Input: part model. Units: mm. Frame: model coordinates. A direction names the side the tool comes from. Give positions to 0.01 mm unless a question says otherwise; leave off trailing zeros. Loops run counter-clockwise (first coordinate to the right, second up) from the corner with the lowest first, then second, coordinate; pieces in that order, holes last. Notation, with made-up numbers: (62, -4.5) - (100, -4.5) arc R20 cw to (100, 5.5) - close; hole circle Ø7 at (68, -24.5). An arc over 180 degrees is marked (long way). Answer as a JSON object with one key per item and string values.
from build123d import *

# Parameters (mm, degrees)
MODEL_R             = 1.6
MODEL_R_2           = 2
BOSS_EXTRUDE1_DEPTH = 10


with BuildPart() as part:
    # Model → Boss-Extrude1 (new body)
    with BuildSketch(Plane.XY):
        Polygon((85, 428), (85, 0), (-85, 0), (-85, 428), (-77, 436), (77, 436), align=None)
        with Locations((-31.5, 50)):
            Circle(MODEL_R, mode=Mode.SUBTRACT)
        with Locations((-31.5, 30)):
            Circle(MODEL_R, mode=Mode.SUBTRACT)
        with Locations((31.5, 30)):
            Circle(MODEL_R, mode=Mode.SUBTRACT)
        with Locations((31.5, 50)):
            Circle(MODEL_R, mode=Mode.SUBTRACT)
        with Locations((-58, 50)):
            Circle(MODEL_R, mode=Mode.SUBTRACT)
        with Locations((-73, 210)):
            Circle(MODEL_R_2, mode=Mode.SUBTRACT)
        with Locations((-73, 230)):
            Circle(MODEL_R_2, mode=Mode.SUBTRACT)
        with Locations((60, 355)):
            Circle(MODEL_R, mode=Mode.SUBTRACT)
        with Locations((58, 50)):
            Circle(MODEL_R, mode=Mode.SUBTRACT)
        with Locations((-60, 355)):
            Circle(MODEL_R, mode=Mode.SUBTRACT)
        with Locations((-28, 355)):
            Circle(MODEL_R, mode=Mode.SUBTRACT)
        with Locations((28, 355)):
            Circle(MODEL_R, mode=Mode.SUBTRACT)
        with Locations((60, 5)):
            Circle(MODEL_R, mode=Mode.SUBTRACT)
        with Locations((28, 5)):
            Circle(MODEL_R, mode=Mode.SUBTRACT)
        with Locations((-28, 5)):
            Circle(MODEL_R, mode=Mode.SUBTRACT)
        with Locations((-60, 5)):
            Circle(MODEL_R, mode=Mode.SUBTRACT)
        with Locations((10, 375)):
            Circle(MODEL_R, mode=Mode.SUBTRACT)
        with Locations((-10, 375)):
            Circle(MODEL_R, mode=Mode.SUBTRACT)
        with BuildLine():
            Line((14, 34.5), (20, 34.5))
            ThreePointArc((20, 34.5), (21.414213562, 33.914213562), (22, 32.5))
            Line((22, 32.5), (22, 14.5))
            ThreePointArc((22, 14.5), (21.414213562, 13.085786438), (20, 12.5))
            Line((20, 12.5), (14, 12.5))
            ThreePointArc((14, 12.5), (12.585786438, 13.085786438), (12, 14.5))
            Line((12, 14.5), (12, 32.5))
            ThreePointArc((12, 32.5), (12.585786438, 33.914213562), (14, 34.5))
        make_face(mode=Mode.SUBTRACT)
        Polygon((-29, 315), (29, 315), (35, 309), (35, 61), (29, 55), (-29, 55), (-35, 61), (-35, 309), align=None, mode=Mode.SUBTRACT)
        with BuildLine():
            Line((-54, 392), (-54, 412))
            ThreePointArc((-54, 412), (-52.242640687, 416.242640687), (-48, 418))
            Line((-48, 418), (48, 418))
            ThreePointArc((48, 418), (52.242640687, 416.242640687), (54, 412))
            Line((54, 412), (54, 392))
            ThreePointArc((54, 392), (52.242640687, 387.757359313), (48, 386))
            Line((48, 386), (-48, 386))
            ThreePointArc((-48, 386), (-52.242640687, 387.757359313), (-54, 392))
        make_face(mode=Mode.SUBTRACT)
    extrude(amount=BOSS_EXTRUDE1_DEPTH)


solid = part.part
Item 1: Cut plane C-C (y = 406.5). Return loops of the section in (x, z), then the cut area to 3 significant figures.
Geometry check:
{"outline": "(-85, 0) - (-54, 0) - (-54, 10) - (-85, 10) - close; (54, 0) - (85, 0) - (85, 10) - (54, 10) - close", "area": "620 mm2"}
Item 2: Mould query, pull axis Y, two halves, no side actions, for faces 3 (the face through (-1, 418, 5)), 4 (the face through (-1, 436, 5)), 5 (the face through (-85, 211, 5)), 6 (the face through (35, 187, 5)). Classes: released by +Y, released by -Y, zero draft, split by the parting line, or undercut.
Geometry check:
{"face 3": "undercut", "face 4": "released by +Y", "face 5": "zero draft", "face 6": "undercut"}
Item 3: Contact query for a flat-ended pin moving along its axis: P1, Ø3, axis at x = 58, y = 50, coming from the +Z side. Output: stop coordinate, or through.
Geometry check:
{"P1": "passes through"}
Item 4: Material intervals for line 1 (Y direction, x = -3, z = 3.25); line 2 (Y direction, x = 13.5, z = 4.5); line 3 (X direction, y = 355, z = 6.5), sorted ascending. Write a range as [from, to].
Geometry check:
{"line 1": "y = [0, 55], [315, 386], [418, 436]", "line 2": "y = [0, 12.56], [34.44, 55], [315, 386], [418, 436]", "line 3": "x = [-85, -61.6], [-58.4, -29.6], [-26.4, 26.4], [29.6, 58.4], [61.6, 85]"}
Item 5: Access query for faces 1 (the face through (-37, 221, 0)), 2 (the face through (0, 315, 5)). Directions: +Z, -Z, +X, -X, +Y, -Y. A direction counts if a zero-diameter tool reaches every point of the face in a straight line with its end or side. Return the directions, or none.
Geometry check:
{"face 1": "-Z, +X, -X, +Y, -Y", "face 2": "+Z, -Z"}
Item 6: Cut plane B-B (z = 5.75). Give the number of separate pieces and of enclosed holes in the cut face, then the cut area to 3 significant figures.
Geometry check:
{"separate pieces": "1", "enclosed holes": "21", "area": "52,100 mm2"}
Item 7: Cut plane A-A (y = 176). Return loops of the section in (x, z), then the cut area to 3 significant figures.
Geometry check:
{"outline": "(-85, 0) - (-35, 0) - (-35, 10) - (-85, 10) - close; (35, 0) - (85, 0) - (85, 10) - (35, 10) - close", "area": "1,000 mm2"}
